Could you check a few things on this model? Use its own coordinates, in mm. A direction names the side the tool comes from. Give positions to 0.01 mm unless a question says otherwise; leave off trailing zeros. Loops run counter-clockwise (first coordinate to the right, second up) from the corner with the lowest first, then second, coordinate; pieces in that order, holes last. Notation, with made-up numbers: (-35.5, 86.5) - (-25.5, 86.5) arc R8 ccw to (-25.5, 94.5) - close; hole circle Ø11 at (-25, 30). An arc over 180 degrees is marked (long way). Write each question's results on one line, items separated by ' | '. Start each with the question number.
```python
from build123d import *

# Parameters (mm, degrees)
F1_DEPTH = 76.2
F3_D     = 6.7564


with BuildPart() as f1:
    # F0 (on Front) → F1 (new body)
    with BuildSketch(Plane.XZ):
        Polygon((0, 2.54), (0, 0), (15.24, 0), (15.24, 50.8), (97.79, 50.8), (97.79, 0), (113.03, 0), (113.03, 2.54), (100.33, 2.54), (100.33, 53.34), (12.7, 53.34), (12.7, 2.54), align=None)
    extrude(amount=-F1_DEPTH)

    # F3 (through all)
    with Locations(Plane.XY.offset(2.54)):
        with Locations((6.35, 63.5), (6.35, 12.7), (106.68, 12.7), (106.68, 63.5)):
            Hole(F3_D / 2)


solid = f1.part
```
Q1. I'm going to push flat-ended pins straight in: pin 1 Ø1 at (y, z) = (30.5, 25) entering from -X; pin 2 Ø9 at (x, y) = (106.68, 63.5) entering from +Z; pin 3 Ø6 at (x, y) = (6.35, 12.7) entering from +Z; pin 4 Ø8 at (y, z) = (19.5, 29.5) entering from +X. Where does each tip first touch, or does it pass through?
Q2. I need wall thicknesses on L1, parallel to Y at x = 6.35, z = 0.7; L2, parallel to X at y = 11.5, z = 43.5; L3, parallel to Y at x = 106, z = 1. Which ranges of each line are inside material? Lowest first, please. Write a range as from..to.
Q3. I want a section at C-C, the plane z = 48.5. List the corners of the cut face in (x, y) for me, then the cut area to 3 significant figures.
Q4. Which directions (+Z, -Z, +X, -X, +Y, -Y) give clear straight access to the entire face, cutting with the end or side of a thin tool? Please do faces 5 (the face through (6, 38, 2.54)), 6 (the face through (100.33, 38, 28)), 7 (the face through (15.24, 38, 25)), 8 (the face through (56, 0, 52)).
Q5. I want a section at D-D, the plane y = 58. List the corners of the cut face in (x, z) for me, then the cut area to 3 significant figures.
Q6. If we mould it in two halves opening along X, with no side actions, what happens to faces 1 (the face through (3.229, 11.406, 1.252)), 2 (the face through (0, 38, 1)), 3 (the face through (57, 38, 53.34)), 4 (the face through (109.361, 61.444, 1.252))? For each: +X half, -X half, draft (parallel to the pull), parting line (faces both ways), or undercut.
Q7. I want a section at A-A, the plane y = 12.7. List the corners of the cut face in (x, z) for me.
Q8. I want a section at B-B, the plane x = 6.35. List the corners of the cut face in (y, z) for me, then the cut area to 3 significant figures.
Conclusion:
1) pin 1: x = 12.7 | pin 2: z = 2.54 | pin 3: through | pin 4: x = 100.33
2) L1: 0..9.32, 16.08..60.12, 66.88..76.2 | L2: 12.7..15.24, 97.79..100.33 | L3: 0..9.39, 16.01..60.19, 66.81..76.2
3) outline: (12.7, 0) - (15.24, 0) - (15.24, 76.2) - (12.7, 76.2) - close; (97.79, 0) - (100.33, 0) - (100.33, 76.2) - (97.79, 76.2) - close | area: 387 mm^2
4) face 5: +Z, -X, +Y, -Y | face 6: +Z, +X, +Y, -Y | face 7: -Z, +Y, -Y | face 8: +Z, -Z, +X, -X, -Y
5) outline: (0, 0) - (15.24, 0) - (15.24, 50.8) - (97.79, 50.8) - (97.79, 0) - (113.03, 0) - (113.03, 2.54) - (100.33, 2.54) - (100.33, 53.34) - (12.7, 53.34) - (12.7, 2.54) - (0, 2.54) - close | area: 545 mm^2
6) face 1: undercut | face 2: -X half | face 3: draft | face 4: undercut
7) outline: (0, 0) - (2.97, 0) - (2.97, 2.54) - (0, 2.54) - close; (9.73, 0) - (15.24, 0) - (15.24, 50.8) - (97.79, 50.8) - (97.79, 0) - (103.3, 0) - (103.3, 2.54) - (100.33, 2.54) - (100.33, 53.34) - (12.7, 53.34) - (12.7, 2.54) - (9.73, 2.54) - close; (110.06, 0) - (113.03, 0) - (113.03, 2.54) - (110.06, 2.54) - close
8) outline: (0, 0) - (9.32, 0) - (9.32, 2.54) - (0, 2.54) - close; (16.08, 0) - (60.12, 0) - (60.12, 2.54) - (16.08, 2.54) - close; (66.88, 0) - (76.2, 0) - (76.2, 2.54) - (66.88, 2.54) - close | area: 159 mm^2
